Verification items for the finished model (mm, model axes). A direction names the side the tool comes from. Coordinates: 2 decimals unless noted, no trailing zeros. Write each loop counter-clockwise with the first axis right and the second up, starting at its lowest first coordinate (ties: lowest second). Pieces come first, ordered by that corner, then holes. Notation, with made-up numbers: M -14,-33.5 L 29,-33.5 A18 ccw 29,1.5 Z; hole C 34.25,-20.5 d8. An arc over 180 degrees is marked long. Answer in a Markdown table with one row per item.
from build123d import *

# Parameters (mm, degrees)
F1_DEPTH = 101.789
F2_W     = 56
F2_H     = 13.3945
F3_DEPTH = 25
F4_R     = 1.6
F5_DEPTH = 15
F6_R     = 0.5


with BuildPart() as f1:
    # F0 (on Front) → F1 (new body)
    with BuildSketch(Plane.XZ):
        Polygon((-80, 0), (0, 0), (0, 6.7567332238), (-80, 18), align=None)
    extrude(amount=F1_DEPTH)

    # F2 (on face) → F3 (cut)
    with BuildSketch(Plane(origin=(0, 0, 0), x_dir=(1, 0, 0), z_dir=(0, 0, -1))):
        with Locations((-40, 70.09175)):
            Rectangle(F2_W, F2_H)
        with Locations((-40, 31.69725)):
            Rectangle(F2_W, F2_H)
    extrude(amount=-F3_DEPTH, mode=Mode.SUBTRACT)

    # F4 (on face) → F5 (cut)
    with BuildSketch(Plane(origin=(0.9312040399, 0, 6.6258610308), x_dir=(0.9902680687, 0, -0.139173101), z_dir=(0.139173101, 0, 0.9902680687))):
        with Locations((-77.9165613166, -3.81)):
            Circle(F4_R)
        with Locations((-77.9165613166, -97.979)):
            Circle(F4_R)
    extrude(amount=-F5_DEPTH, mode=Mode.SUBTRACT)

    # F6
    f6_edges = [f1.edges().sort_by_distance(p)[0] for p in [
        (-77.811508, -97.979, 17.692427),
        (-77.811508, -3.81, 17.692427),
        (-80, -50.8945, 0),
        (-40, 0, 0),
        (-40, -101.789, 0),
        (0, -50.8945, 0),
        (-12, -70.09175, 0),
        (-40, -63.3945, 0),
        (-68, -70.09175, 0),
        (-40, -76.789, 0),
        (-40, -25, 0),
        (-68, -31.69725, 0),
        (-40, -38.3945, 0),
        (-12, -31.69725, 0),
    ]]
    fillet(f6_edges, radius=F6_R)


solid = f1.part
1) Thickness scan on L1, parallel to Y at x = -38.5, z = 4.25; L2, parallel to X at y = -27, z = 6.5; L3, parallel to X at y = -31, z = 15.25. Record the ranges inside material, lowest first. Write a range as [from, to].
Response values:
| item | result |
|---|---|
| L1 | y = [-101.79, -76.79], [-63.39, -38.39], [-25, 0] |
| L2 | x = [-80, -68], [-12, 0] |
| L3 | x = [-80, -68] |
2) Sectioned sample at A-A (y = -28). Record the cut outline in (x, z), then the cut area to 3 significant figures.
Response values:
| item | result |
|---|---|
| outline | M -80,0.5 A0.5 ccw -79.5,0 L -68.5,0 A0.5 ccw -68,0.5 L -68,16.31 L -80,18 Z; M -12,0.5 A0.5 ccw -11.5,0 L -0.5,0 A0.5 ccw 0,0.5 L 0,6.76 L -12,8.44 Z |
| area | 297 mm² |
3) Sectioned sample at D-D (z = 14). Give the number of separate pieces and of enclosed holes in the cut face, then the cut area to 3 significant figures.
Response values:
| item | result |
|---|---|
| separate pieces | 1 |
| enclosed holes | 2 |
| area | 2,440 mm² |
4) Sectioned sample at C-C (y = -11). Record the cut outline in (x, z).
Response values:
| item | result |
|---|---|
| outline | M -80,0.5 A0.5 ccw -79.5,0 L -0.5,0 A0.5 ccw 0,0.5 L 0,6.76 L -80,18 Z |
5) Depth check by flat-ended pin: pin 1 (4 mm diameter, centred on y = -82.5, z = 8.5, fed in from +X). Enter the tip coordinate at first touch or a pass-through.
Response values:
| item | result |
|---|---|
| pin 1 | stops at x = 0 |
6) Tool access check on faces 1 (the face through (-49, -101.789, 7)), 2 (the face through (-12, -32, 4)), 3 (the face through (-78.34, -3.79, 2.62)). Record the directions out of +Z, -Z, +X, -X, +Y, -Y that give a thin tool (end or side, any length) a straight path to the whole face; none if there is none.
Response values:
| item | result |
|---|---|
| face 1 | +Z, -Z, +X, -X, -Y |
| face 2 | +Z, -Z |
| face 3 | none |
7) Release check for a two-part mould opening along Z. For faces 4 (the face through (-41, -50, 0)), 5 (the face through (-68, -32, 8)), 6 (the face through (-77.64, -99.54, 9.94)) record: +Z half, -Z half, draft (parallel to the pull), parting line (faces both ways), or undercut.
Response values:
| item | result |
|---|---|
| face 4 | -Z half |
| face 5 | draft |
| face 6 | undercut |
8) Sectioned sample at B-B (x = -62). Record the cut outline in (y, z), then the cut area to 3 significant figures.
Response values:
| item | result |
|---|---|
| outline | M -101.79,0.5 A0.5 ccw -101.29,0 L -77.29,0 A0.5 ccw -76.79,0.5 L -76.79,15.47 L -101.79,15.47 Z; M -63.39,0.5 A0.5 ccw -62.89,0 L -38.89,0 A0.5 ccw -38.39,0.5 L -38.39,15.47 L -63.39,15.47 Z; M -25,0.5 A0.5 ccw -24.5,0 L -0.5,0 A0.5 ccw 0,0.5 L 0,15.47 L -25,15.47 Z |
| area | 1,160 mm² |
